```python
from build123d import *

# Parameters (mm, degrees)
SKETCH1_W           = 196.85
SKETCH1_H           = 101.6
SKETCH1_R           = 3.429
SKETCH1_W_2         = 133.35
SKETCH1_H_2         = 88.9
BOSS_EXTRUDE1_DEPTH = 6.35


with BuildPart() as part:
    # Sketch1 → Boss-Extrude1 (new body)
    with BuildSketch(Plane(origin=(0, 0, 0), x_dir=(1, 0, 0), z_dir=(0, 1, 0))):
        Rectangle(SKETCH1_W, SKETCH1_H)
        with Locations(Location((-85.725, 38.1, 0), (0, 0, 270))):
            Circle(SKETCH1_R, mode=Mode.SUBTRACT)
        with Locations(Location((85.725, 38.1, 0), (0, 0, 270))):
            Circle(SKETCH1_R, mode=Mode.SUBTRACT)
        with Locations(Location((85.725, 25.4, 0), (0, 0, 270))):
            Circle(SKETCH1_R, mode=Mode.SUBTRACT)
        with Locations(Location((85.725, 12.7, 0), (0, 0, 270))):
            Circle(SKETCH1_R, mode=Mode.SUBTRACT)
        with Locations(Location((85.725, 0, 0), (0, 0, 270))):
            Circle(SKETCH1_R, mode=Mode.SUBTRACT)
        with Locations(Location((85.725, -12.7, 0), (0, 0, 270))):
            Circle(SKETCH1_R, mode=Mode.SUBTRACT)
        with Locations(Location((85.725, -25.4, 0), (0, 0, 270))):
            Circle(SKETCH1_R, mode=Mode.SUBTRACT)
        with Locations(Location((85.725, -38.1, 0), (0, 0, 270))):
            Circle(SKETCH1_R, mode=Mode.SUBTRACT)
        with Locations(Location((-85.725, 25.4, 0), (0, 0, 270))):
            Circle(SKETCH1_R, mode=Mode.SUBTRACT)
        with Locations(Location((-85.725, 12.7, 0), (0, 0, 270))):
            Circle(SKETCH1_R, mode=Mode.SUBTRACT)
        with Locations(Location((-85.725, 0, 0), (0, 0, 270))):
            Circle(SKETCH1_R, mode=Mode.SUBTRACT)
        with Locations(Location((-85.725, -12.7, 0), (0, 0, 270))):
            Circle(SKETCH1_R, mode=Mode.SUBTRACT)
        with Locations(Location((-85.725, -25.4, 0), (0, 0, 270))):
            Circle(SKETCH1_R, mode=Mode.SUBTRACT)
        with Locations(Location((-85.725, -38.1, 0), (0, 0, 270))):
            Circle(SKETCH1_R, mode=Mode.SUBTRACT)
        Rectangle(SKETCH1_W_2, SKETCH1_H_2, mode=Mode.SUBTRACT)
    extrude(amount=BOSS_EXTRUDE1_DEPTH)


solid = part.part
```
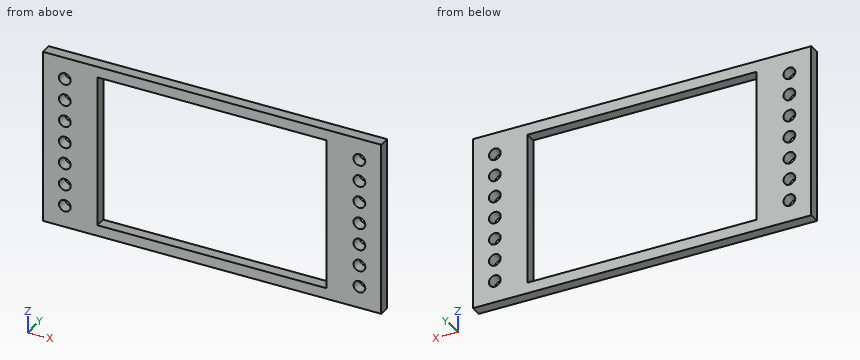
For this review, take the finished solid that the model builds, in its own axes (mm). Coordinates: 2 decimals unless noted, no trailing zeros. Loops run counter-clockwise (first coordinate to the right, second up) from the corner with the lowest first, then second, coordinate; pieces in that order, holes last. Notation, with made-up numbers: (41, 75.5) -> (91, 75.5) arc R21 cw to (91, 89.5) -> close; hole circle Ø1 at (74, -17.75). An arc over 180 degrees is marked (long way). Return JSON: item names as keys, results as strings. Group by question number.
(1) Consider section B-B, the plane x = -46. Give the boundary of the cut face in (y, z).
(2) Consider section A-A, the plane z = 0. Give the boundary of the cut face in (x, y) (3 decimals).
(3) Consider section C-C, the plane z = 19. Give the boundary of the cut face in (x, y) (3 decimals).
(4) For pin 1 Ø8 at (x, z) = (-85.725, 25.4) entering from -Y; pin 2 Ø5.5 at (x, z) = (-85.725, 0) entering from -Y, all flat-tipped, find the tip position at first contact; note any pin that passes through.
(5) Consider section D-D, the plane y = 4.5. Count the separate pieces of the cut face and the enclosed holes in it, plus the area to 3 significant figures.
(6) To check wall thickness, follow L1, parallel to X at y = 2.5, z = 0 (3 decimals); L2, parallel to Z at x = 44, y = 2.5; L3, parallel to X at y = 0.5, z = 14 (3 decimals). State the ranges of each line that lie inside material, in increasing order.
Results below:
{
 "1": {"outline": "(0, -50.8) -> (6.35, -50.8) -> (6.35, -44.45) -> (0, -44.45) -> close; (0, 44.45) -> (6.35, 44.45) -> (6.35, 50.8) -> (0, 50.8) -> close"},
 "2": {"outline": "(-98.425, 0) -> (-89.154, 0) -> (-89.154, 6.35) -> (-98.425, 6.35) -> close; (-82.296, 0) -> (-66.675, 0) -> (-66.675, 6.35) -> (-82.296, 6.35) -> close; (66.675, 0) -> (82.296, 0) -> (82.296, 6.35) -> (66.675, 6.35) -> close; (89.154, 0) -> (98.425, 0) -> (98.425, 6.35) -> (89.154, 6.35) -> close"},
 "3": {"outline": "(-98.425, 0) -> (-66.675, 0) -> (-66.675, 6.35) -> (-98.425, 6.35) -> close; (66.675, 0) -> (98.425, 0) -> (98.425, 6.35) -> (66.675, 6.35) -> close"},
 "4": {"pin 1": "stops at y = 0", "pin 2": "passes through"},
 "5": {"separate pieces": "1", "enclosed holes": "15", "area": "7,630 mm2"},
 "6": {"L1": "x = -98.425 to -89.154, -82.296 to -66.675, 66.675 to 82.296, 89.154 to 98.425", "L2": "z = -50.8 to -44.45, 44.45 to 50.8", "L3": "x = -98.425 to -88.898, -82.552 to -66.675, 66.675 to 82.552, 88.898 to 98.425"}
}
